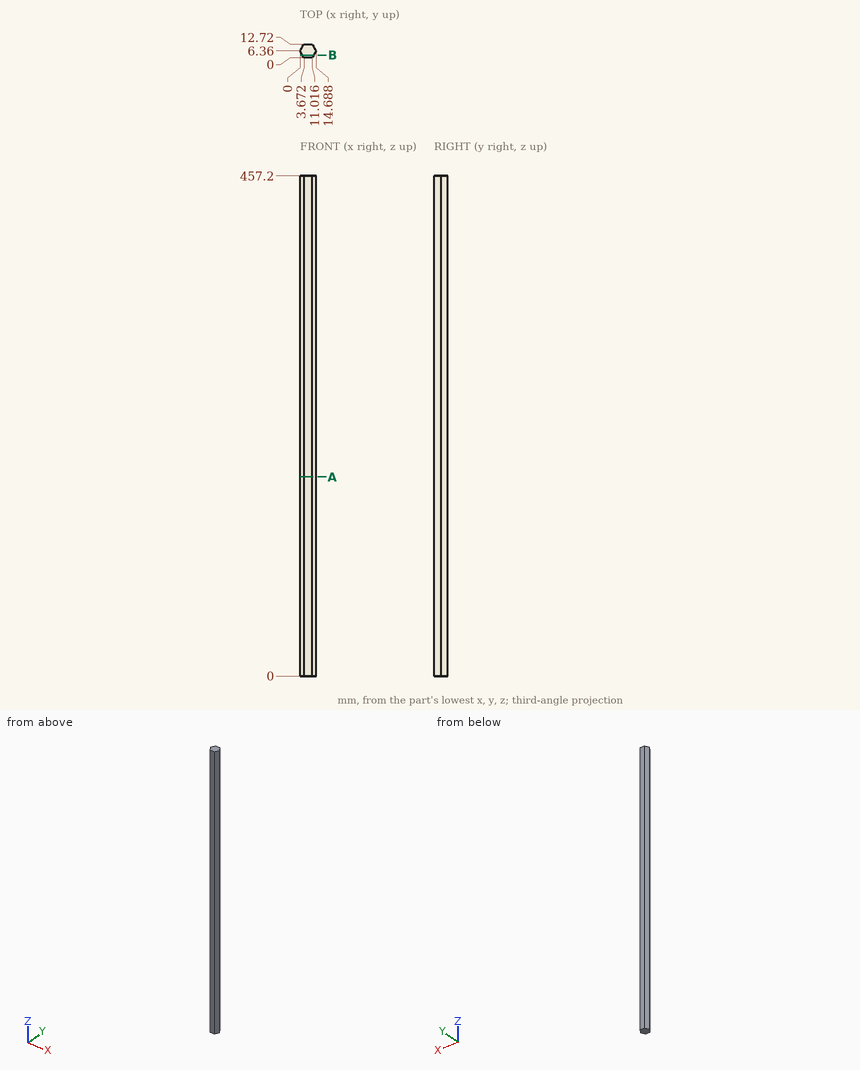
Study the drawing (mm; zero at the part's minimum x, y, z) and answer. Give positions to 0.01 mm unless a question says otherwise; leave off trailing zeros. Write each loop counter-clockwise with the first axis right and the second up, starting at its lowest first coordinate (ties: lowest second). Pieces come first, ordered by that corner, then holes. Notation, with made-up numbers: (3.25, -5) - (29.25, -5) arc R14 cw to (29.25, 20) - close; hole circle Ø1 at (-7, 11). An arc over 180 degrees is marked (long way). Write item = value, one per line. Start each with the question number.
Item 1: Find section B-B (y = 2.5). Give the vertices of the cut face in (x, z), then the cut area to 3 significant figures.
Item 2: Each of these flat-tipped pins is pushed along its axis until it touches: P1, Ø1.5, axis at y = 3.5, z = 399.5, coming from the -X side; P2, Ø8, axis at x = 11.5, z = 94, coming from the -Y side; P3, Ø1, axis at y = 2.5, z = 407, coming from the -X side. Where does it stop, or does it pass through?
Item 3: Find section A-A (z = 182). Give the vertices of the cut face in (x, y).
Item 4: Find the intervals of material crossed by probe 1 along X at (y, z) = (6.25, 331) (1 decimal); probe 2 along X at (y, z) = (2.5, 139); probe 3 along Y at (x, z) = (3.5, 218.5), in increasing order. Write a range as [from, to].
Response:
q1.outline = (2.23, 0) - (12.46, 0) - (12.46, 457.2) - (2.23, 457.2) - close
q1.area = 4,680 mm²
q2.P1 = 1.22
q2.P2 = 0
q2.P3 = 1.94
q3.outline = (0, 6.36) - (3.67, 0) - (11.02, 0) - (14.69, 6.36) - (11.02, 12.72) - (3.67, 12.72) - close
q4.probe_1 = [0.1, 14.6]
q4.probe_2 = [2.23, 12.46]
q4.probe_3 = [0.3, 12.42]
